Could you check a few things on this model? Use its own coordinates, in mm. Round coordinates to 2 decimals unless told otherwise and drop trailing zeros. Write each loop counter-clockwise with the first axis right and the second up, starting at its lowest first coordinate (ties: lowest second). Pieces come first, ordered by that corner, then holes. Notation, with made-up numbers: (8.25, -0.5) -> (14.25, -0.5) arc R21 ccw to (14.25, 5.5) -> close; hole circle Ø6 at (29.5, -12). An arc over 180 degrees is marked (long way). One line per question, with ' | ' between items. Start each with the question number.
1. If I drill on line 1 along X through (y, z) = (-16.75, 38); line 2 along Z through (x, y) = (-38.5, -7.5); line 3 along X through (y, z) = (-2.75, 32.5), over which ranges is the centre line in solid material (lowest first)? Write a range as [from, to].
2. For pin 1 Ø12 at (x, y) = (-48, -8) entering from -Z; pin 2 Ø11.5 at (x, z) = (-37.96, 62.88) entering from -Y, each with a flat end and sliding along its axis, tell me the tip position at first contact or that it passes through.
3. Thinking about a two-plate mould opening in X: for faces 1 (the flat face through (-39, -13, 0)), 2 (the cylindrical face through (-69.708, -12.878, 37.76)), 3 (the flat face through (-76.064, -13, 37)), which applies, released by +X, released by -X, zero draft, split by the parting line, or undercut?
4. Imagine slicing it at D-D, the plane x = -37.5. List the corners of the cut face in (y, z) for me, and give its area (3 significant figures).
5. Imagine slicing it at C-C, the plane z = 59. List the corners of the cut face in (x, y) for me, and give its area (3 significant figures).
6. Imagine slicing it at A-A, the plane x = -46.5. List the corners of the cut face in (y, z) for me, and give its area (3 significant figures).
7. Imagine slicing it at B-B, the plane y = -6.25. List the corners of the cut face in (x, z) for me.
from build123d import *

# Parameters (mm, degrees)
F0_W     = 76.064058
F0_H     = 75.58123
F1_DEPTH = 25.4
F2_R     = 12.7
F3_DEPTH = 25.401
F4_R     = 6.35
F5_DEPTH = 25.401


with BuildPart() as f1:
    # F0 (on Front) → F1 (new body)
    with BuildSketch(Plane.XZ):
        with Locations((-38.032029, 37.790615)):
            Rectangle(F0_W, F0_H)
    extrude(amount=F1_DEPTH)

    # F2 (on face) → F3 (cut, through all)
    with BuildSketch(Plane(origin=(0, 0, 0), x_dir=(-1, 0, 0), z_dir=(0, 1, 0))):
        with Locations((37.964058, 37.48123)):
            Circle(F2_R)
    extrude(amount=-F3_DEPTH, mode=Mode.SUBTRACT)

    # F4 (on face) → F5 (cut, through all)
    with BuildSketch(Plane.XZ.offset(25.4)):
        with Locations((-37.964058, 62.88123)):
            Circle(F4_R)
        with Locations((-63.364058, 37.48123)):
            Circle(F4_R)
        with Locations((-37.964058, 12.08123)):
            Circle(F4_R)
        with Locations((-12.564058, 37.48123)):
            Circle(F4_R)
    extrude(amount=-F5_DEPTH, mode=Mode.SUBTRACT)


solid = f1.part
Geometry results:
1) line 1: x = [-76.06, -69.69], [-57.04, -50.65], [-25.27, -18.89], [-6.24, 0] | line 2: z = [0, 5.75], [18.41, 24.79], [50.17, 56.55], [69.21, 75.58] | line 3: x = [-76.06, -67.3], [-59.43, -49.65], [-26.28, -16.5], [-8.63, 0]
2) pin 1: stops at z = 0 | pin 2: passes through
3) face 1: zero draft | face 2: undercut | face 3: released by -X
4) outline: (-25.4, 0) -> (0, 0) -> (0, 5.75) -> (-25.4, 5.75) -> close; (-25.4, 18.41) -> (0, 18.41) -> (0, 24.79) -> (-25.4, 24.79) -> close; (-25.4, 50.17) -> (0, 50.17) -> (0, 56.55) -> (-25.4, 56.55) -> close; (-25.4, 69.21) -> (0, 69.21) -> (0, 75.58) -> (-25.4, 75.58) -> close | area: 632 mm2
5) outline: (-76.06, -25.4) -> (-42.99, -25.4) -> (-42.99, 0) -> (-76.06, 0) -> close; (-32.94, -25.4) -> (0, -25.4) -> (0, 0) -> (-32.94, 0) -> close | area: 1,680 mm2
6) outline: (-25.4, 0) -> (0, 0) -> (0, 28.08) -> (-25.4, 28.08) -> close; (-25.4, 46.88) -> (0, 46.88) -> (0, 75.58) -> (-25.4, 75.58) -> close | area: 1,440 mm2
7) outline: (-76.06, 0) -> (0, 0) -> (0, 75.58) -> (-76.06, 75.58) -> close; hole circle Ø12.7 at (-63.36, 37.48); hole circle Ø25.4 at (-37.96, 37.48); hole circle Ø12.7 at (-37.96, 12.08); hole circle Ø12.7 at (-37.96, 62.88); hole circle Ø12.7 at (-12.56, 37.48)
